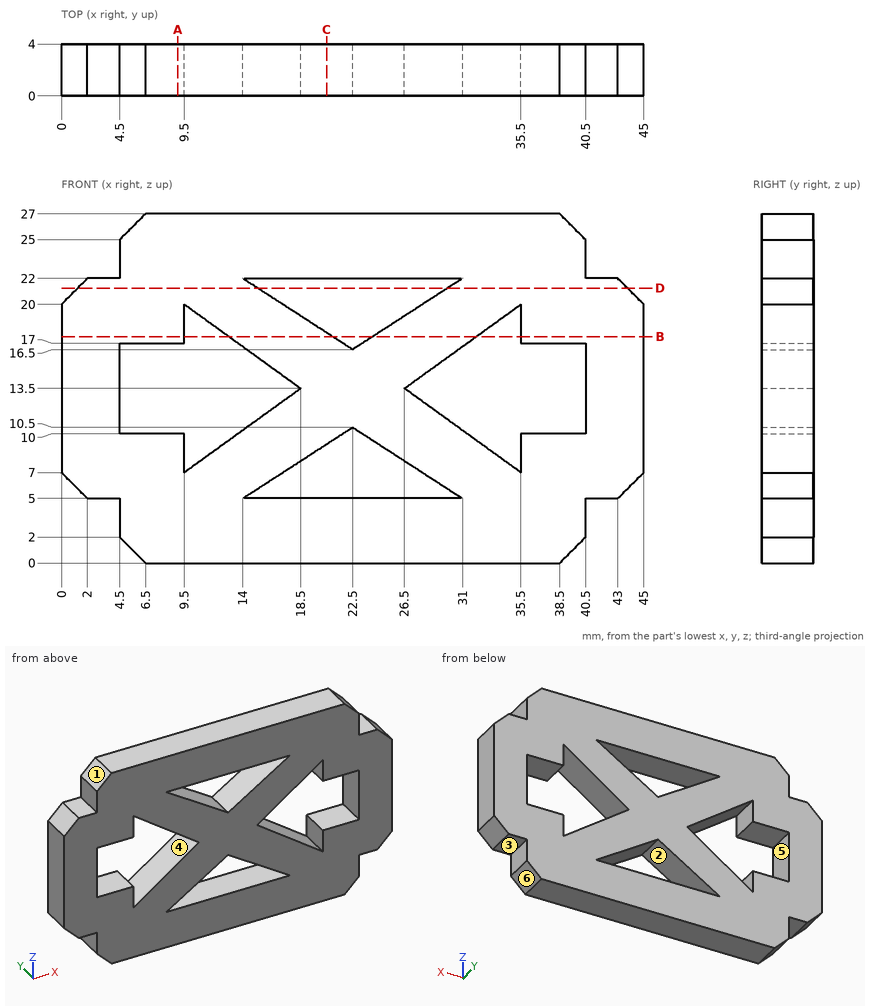
Study the drawing (mm; zero at the part's minimum x, y, z) and answer. A direction names the side the tool comes from. Give positions to 0.01 mm unless a question says otherwise; leave off trailing zeros. Write each loop counter-clockwise with the first axis right and the second up, starting at its lowest first coordinate (ties: lowest second). Pieces come first, ordered by that corner, then holes. Notation, with made-up numbers: (-32.75, -8) -> (-16.75, -8) arc R19 ccw to (-16.75, 20) -> close; hole circle Ø5 at (-27, 36.5). An arc over 180 degrees is marked (long way). Answer in a Markdown table with one row per item.
1) Section D-D on z = 21.25 is taken. Give the vertices of the cut face in (x, y).
Results list:
| item | result |
|---|---|
| outline | (1.25, 0) -> (15.16, 0) -> (15.16, 4) -> (1.25, 4) -> close; (29.84, 0) -> (43.75, 0) -> (43.75, 4) -> (29.84, 4) -> close |
2) Each of these flat-tipped pins is pushed along its axis until it touches: pin 1 Ø1.2 at (x, y) = (41.5, 1) entering from -Z; pin 2 Ø1 at (y, z) = (3, 24) entering from -X; pin 3 Ø1.2 at (x, y) = (4, 1.5) entering from -Z. Where does it stop, or does it pass through?
Results list:
| item | result |
|---|---|
| pin 1 | z = 5 |
| pin 2 | x = 4.5 |
| pin 3 | z = 1.9 |
3) Section C-C on x = 20.5 is taken. Give the vertices of the cut face in (y, z), plus the area to 3 significant figures.
Results list:
| item | result |
|---|---|
| outline | (0, 0) -> (4, 0) -> (4, 5) -> (0, 5) -> close; (0, 9.21) -> (4, 9.21) -> (4, 17.79) -> (0, 17.79) -> close; (0, 22) -> (4, 22) -> (4, 27) -> (0, 27) -> close |
| area | 74.4 mm^2 |
4) Straight lines are drawn through the part: line 1 (Z direction, x = 26, y = 1.95); line 2 (Z direction, x = 29, y = 1.15); line 3 (Z direction, x = 17.5, y = 2.5). For each, find the intervals that lie inside material, in ascending order. Write a range as [from, to].
Results list:
| item | result |
|---|---|
| line 1 | [0, 5], [8.24, 18.76], [22, 27] |
| line 2 | [0, 5], [6.29, 11.69], [15.31, 20.71], [22, 27] |
| line 3 | [0, 5], [7.26, 12.78], [14.22, 19.74], [22, 27] |
5) Section A-A on x = 9 is taken. Give the vertices of the cut face in (y, z), plus the area to 3 significant figures.
Results list:
| item | result |
|---|---|
| outline | (0, 0) -> (4, 0) -> (4, 10) -> (0, 10) -> close; (0, 17) -> (4, 17) -> (4, 27) -> (0, 27) -> close |
| area | 80.0 mm^2 |
6) Determine the mould class of the marked faces 1, 2, 3 and 4 for opening direction X: released by +X, released by -X, zero draft, split by the parting line, or undercut.
Results list:
| item | result |
|---|---|
| face 1 | released by -X |
| face 2 | undercut |
| face 3 | zero draft |
| face 4 | undercut |
7) A tool of negligible diameter and unlimited length cuts with its end or side. For the marked faces 5 and 6, from which of +Z, -Z, +X, -X, +Y, -Y can it reach the whole face along a straight path? Write none if from no direction.
Results list:
| item | result |
|---|---|
| face 5 | +Y, -Y |
| face 6 | -Z, +X, +Y, -Y |
8) Section B-B on z = 17.5 is taken. Give the vertices of the cut face in (x, y), plus the area to 3 significant figures.
Results list:
| item | result |
|---|---|
| outline | (0, 0) -> (9.5, 0) -> (9.5, 4) -> (0, 4) -> close; (12.96, 0) -> (20.95, 0) -> (20.95, 4) -> (12.96, 4) -> close; (24.05, 0) -> (32.04, 0) -> (32.04, 4) -> (24.05, 4) -> close; (35.5, 0) -> (45, 0) -> (45, 4) -> (35.5, 4) -> close |
| area | 140 mm^2 |
